Part model, mm, in its own coordinate system. A direction names the side the tool comes from. Round coordinates to 2 decimals unless told otherwise and drop trailing zeros. Loops run counter-clockwise (first coordinate to the right, second up) from the corner with the lowest first, then second, coordinate; pieces in that order, holes last. Notation, with made-up numbers: (-24, 24.25) -> (-19, 24.25) arc R20 cw to (-19, 56.25) -> close; hole circle Ø7 at (-19.5, -2.5). An arc over 180 degrees is marked (long way). Answer as a JSON object with one key per item and string values. Group by question number.
from build123d import *

# Parameters (mm, degrees)
ESQUISSE1_W             = 6
ESQUISSE1_H             = 20
ESQUISSE1_W_2           = 30
ESQUISSE1_H_2           = 30
BOSS_EXTRU_1_DEPTH      = 6
ESQUISSE2_W             = 15
ESQUISSE2_H             = 6
ESQUISSE2_W_2           = 6
ESQUISSE2_H_2           = 15
ESQUISSE2_W_3           = 20
BOSS_EXTRU_2_DEPTH      = 6
ESQUISSE3_R             = 1
ESQUISSE3_R_2           = 1.5
ENL_V_MAT_EXTRU_1_DEPTH = 6
ESQUISSE4_W             = 30
ESQUISSE4_H             = 15
ENL_V_MAT_EXTRU_2_DEPTH = 6


with BuildPart() as part:
    # Esquisse1 → Boss.-Extru.1 (new body)
    with BuildSketch(Plane.XY):
        Polygon((-159, 35), (-131, 35), (-131, 62.75), (131, 62.75), (131, 35), (159, 35), (159, -60), (-159, -60), align=None)
        with Locations((93, 37.75)):
            Rectangle(ESQUISSE1_W, ESQUISSE1_H, mode=Mode.SUBTRACT)
        with Locations((93, -35.01)):
            Rectangle(ESQUISSE1_W, ESQUISSE1_H, mode=Mode.SUBTRACT)
        with Locations((-83, 37.75)):
            Rectangle(ESQUISSE1_W, ESQUISSE1_H, mode=Mode.SUBTRACT)
        with Locations((-83, -35.01)):
            Rectangle(ESQUISSE1_W, ESQUISSE1_H, mode=Mode.SUBTRACT)
        with Locations((-110.986534361, 11.825583908)):
            Rectangle(ESQUISSE1_W_2, ESQUISSE1_H_2, mode=Mode.SUBTRACT)
    extrude(amount=BOSS_EXTRU_1_DEPTH)

    # Esquisse2 → Boss.-Extru.2 (add)
    with BuildSketch(Plane.XY.offset(6)):
        with Locations((-85, -63)):
            Rectangle(ESQUISSE2_W, ESQUISSE2_H)
        with Locations((0, -63)):
            Rectangle(ESQUISSE2_W, ESQUISSE2_H)
        with Locations((85, -63)):
            Rectangle(ESQUISSE2_W, ESQUISSE2_H)
        with Locations((-162, 13.59)):
            Rectangle(ESQUISSE2_W_2, ESQUISSE2_H_2)
        with Locations((-162, -31.41)):
            Rectangle(ESQUISSE2_W_2, ESQUISSE2_H_2)
        with Locations((162, -31.41)):
            Rectangle(ESQUISSE2_W_2, ESQUISSE2_H_2)
        with Locations((162, 13.59)):
            Rectangle(ESQUISSE2_W_2, ESQUISSE2_H_2)
        with Locations((91, 65.75)):
            Rectangle(ESQUISSE2_W_3, ESQUISSE2_H)
        with Locations((-91, 65.75)):
            Rectangle(ESQUISSE2_W_3, ESQUISSE2_H)
        with Locations((0, 65.75)):
            Rectangle(ESQUISSE2_W_3, ESQUISSE2_H)
    extrude(amount=-BOSS_EXTRU_2_DEPTH)

    # Esquisse3 → Enlèv. mat.-Extru.1 (cut)
    with BuildSketch(Plane(origin=(0, 0, 0), x_dir=(-1, 0, 0), z_dir=(0, 0, -1))):
        with Locations((138, -31.49)):
            Circle(ESQUISSE3_R)
        with Locations((138, -15.49)):
            Circle(ESQUISSE3_R)
        with Locations((122, -15.49)):
            Circle(ESQUISSE3_R)
        with Locations((122, -31.49)):
            Circle(ESQUISSE3_R)
        with Locations((-122, -31.49)):
            Circle(ESQUISSE3_R)
        with Locations((-122, -15.49)):
            Circle(ESQUISSE3_R)
        with Locations((-138, -15.49)):
            Circle(ESQUISSE3_R)
        with Locations((-138, -31.49)):
            Circle(ESQUISSE3_R)
        with Locations((83, 22.75)):
            Circle(ESQUISSE3_R_2)
        with Locations((83, -20.01)):
            Circle(ESQUISSE3_R_2)
        with Locations((-93, 22.75)):
            Circle(ESQUISSE3_R_2)
        with Locations((-93, -20.01)):
            Circle(ESQUISSE3_R_2)
    extrude(amount=-ENL_V_MAT_EXTRU_1_DEPTH, mode=Mode.SUBTRACT)

    # Esquisse4 → Enlèv. mat.-Extru.2 (cut)
    with BuildSketch(Plane(origin=(0, 0, 0), x_dir=(-1, 0, 0), z_dir=(0, 0, -1))):
        with Locations((45.5, 55.25)):
            Rectangle(ESQUISSE4_W, ESQUISSE4_H)
    extrude(amount=-ENL_V_MAT_EXTRU_2_DEPTH, mode=Mode.SUBTRACT)


solid = part.part
Item 1: Which spindle directions (+Z, -Z, +X, -X, +Y, -Y) get a long thin tool onto all of the face, cutting with end or side? Do faces 1 (the face through (-7.5, -63, 3)), 2 (the face through (159, 28, 3)), 3 (the face through (96, 38, 3)), 4 (the face through (-131, 49, 3)), 5 (the face through (162, -38.91, 3)). Say none if no direction does.
Item 2: Band-saw the part on C-C, the plane x = 26.5. List the corners of the cut face in (y, z), plus the area to 4 significant figures.
Item 3: Drop flat-ended pins along their axis: pin 1 Ø1.8 at (x, z) = (-20, 2.5) entering from +Y; pin 2 Ø1 at (y, z) = (30, 3.5) entering from +X; pin 3 Ø3 at (y, z) = (23.5, 5) entering from -X. Give the stop position or say it passes through.
Item 4: Drill centre lines: line 1 (X direction, y = 43, z = 1.4); line 2 (X direction, y = 34.5, z = 5.35); line 3 (Y direction, x = -122, z = 2.5). Where is each one in solid material? Low to high.
Item 5: Band-saw the part on B-B, the plane y = -9. List the corners of the cut face in (x, z).
Item 6: Two-plate mould, pull along X, no slides. Class faces 6 (the face through (159, -9, 3)), 7 (the face through (0, 68.75, 3)), 8 (the face through (-80, 38, 3)): pulls with the +X half, pulls with the -X half, needs draft (parallel to the pull), parting line crosses it, or undercut.
Item 7: Band-saw the part on A-A, the plane z = 4.7. Count the separate pieces of the cut face and the enclosed holes in it, plus the area to 3 significant figures.
Entries:
{
 "1": {"face 1": "+Z, -Z, -Y", "face 2": "+Z, -Z, +X, +Y", "face 3": "+Z, -Z", "face 4": "+Z, -Z, -X, +Y", "face 5": "+Z, -Z, +X, -Y"},
 "2": {"outline": "(-60, 0) -> (62.75, 0) -> (62.75, 6) -> (-60, 6) -> close", "area": "736.5 mm²"},
 "3": {"pin 1": "y = 62.75", "pin 2": "x = 159", "pin 3": "x = -159"},
 "4": {"line 1": "-131 to -86, -80 to 90, 96 to 131", "line 2": "-159 to -86, -80 to 90, 96 to 159", "line 3": "-60 to -32.49, -30.49 to -16.49, -14.49 to -3.17, 26.83 to 62.75"},
 "5": {"outline": "(-159, 0) -> (159, 0) -> (159, 6) -> (-159, 6) -> close"},
 "6": {"face 6": "pulls with the +X half", "face 7": "needs draft", "face 8": "undercut"},
 "7": {"separate pieces": "1", "enclosed holes": "17", "area": "36,600 mm²"}
}
